Check sheet for the modelled part. Datum: model origin and axes. Units: mm. Coordinates: 2 decimals unless noted, no trailing zeros. Loops run counter-clockwise (first coordinate to the right, second up) from the corner with the lowest first, then second, coordinate; pieces in that order, holes last. Notation, with made-up numbers: (24, 45) -> (78, 45) arc R35 ccw to (78, 79) -> close; hole circle Ø7 at (11, -34.5). An arc over 180 degrees is marked (long way). Use CSV: the item, a comma, the result in double quotes. Start each with the question number.
1. Sectioned sample at C-C, the plane y = 9.5. Record the cut outline in (x, z), and give its area (3 significant figures).
2. Thickness scan on L1, parallel to Y at x = 0, z = 0.1; L2, parallel to Y at x = 0.3, z = 0.3; L3, parallel to Z at x = 0.05, y = 9.75. Record the ranges inside material, lowest first.
3. Sectioned sample at B-B, the plane y = 5.5. Record the cut outline in (x, z) (3 decimals), and give its area (3 significant figures).
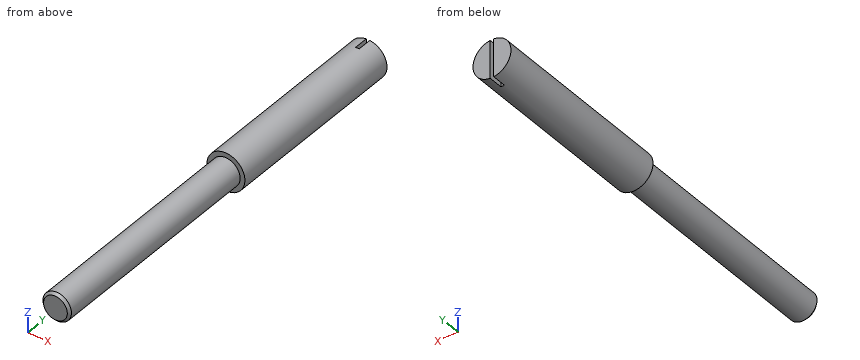
```python
from build123d import *

# Parameters (mm, degrees)
SKETCH2_W               = 0.093
SKETCH2_H               = 0.722554603
CUT_EXTRUDE1_DEPTH      = 1.5
CUT_EXTRUDE1_DEPTH_BACK = 1.5
CHAMFER1_SIZE           = 0.062


with BuildPart() as part:
    # Sketch1 → Revolve1 (revolve)
    with BuildSketch(Plane.XY):
        Polygon((0, 0), (0.375, 0), (0.375, 6), (0.5, 6), (0.5, 11), (0, 11), align=None)
    revolve(axis=Axis((0, -1.490059703, 0), (0, 1, 0)))

    # Sketch2 → Cut-Extrude1 (cut, two sides)
    with BuildSketch(Plane.XY) as cut_extrude1_sk:
        with Locations((0, 10.987009479)):
            Rectangle(SKETCH2_W, SKETCH2_H)
    extrude(amount=CUT_EXTRUDE1_DEPTH, mode=Mode.SUBTRACT)
    extrude(cut_extrude1_sk.sketch, amount=-CUT_EXTRUDE1_DEPTH_BACK, mode=Mode.SUBTRACT)

    # Chamfer1
    chamfer1_edges = [part.edges().sort_by_distance(p)[0] for p in [
        (-0.375, 0, 0),
    ]]
    chamfer(chamfer1_edges, length=CHAMFER1_SIZE)


solid = part.part
```
Completed:
1,outline,"circle Ø1 at (0, 0)"
1,area,"0.785 mm²"
2,L1,"0 to 10.63"
2,L2,"6 to 11"
2,L3,"-0.5 to 0.5"
3,outline,"circle Ø0.75 at (0, 0)"
3,area,"0.442 mm²"
